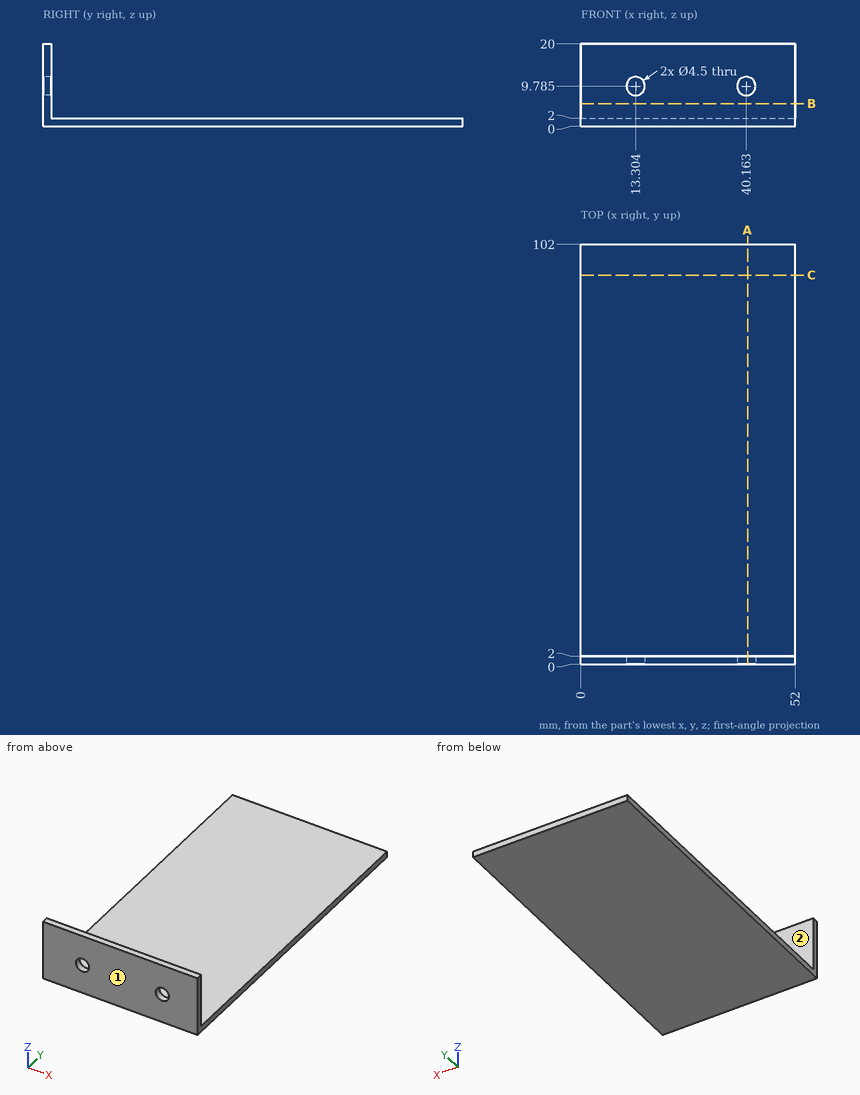
Design review of the part shown in the three views and the two pictorial views. Dimensions are in mm from the part's minimum x, y and z. A direction names the side the tool comes from. Give positions to 0.01 mm unless a question says otherwise; leave off trailing zeros. Loops run counter-clockwise (first coordinate to the right, second up) from the corner with the lowest first, then second, coordinate; pieces in that order, holes last. Notation, with made-up numbers: (8, 6) -> (17, 6) arc R19 ccw to (17, 26) -> close; hole circle Ø4 at (88.25, 33.25). An arc over 180 degrees is marked (long way). One line per item, written item: value.
Q1. We need section A-A on x = 40.5. Give the boundary of the cut face in (y, z), and give its area (3 significant figures).
Numbers:
outline: (0, 0) -> (102, 0) -> (102, 2) -> (2, 2) -> (2, 7.56) -> (0, 7.56) -> close; (0, 12.01) -> (2, 12.01) -> (2, 20) -> (0, 20) -> close
area: 231 mm^2
Q2. For L1, parallel to Z at x = 30, y = 29.5, list the stretches that pass through material, from the lowest coordinate up.
Numbers:
L1: z = 0 to 2
Q3. We need section B-B on z = 5.5. Give the boundary of the cut face in (x, y), and give its area (3 significant figures).
Numbers:
outline: (0, 0) -> (52, 0) -> (52, 2) -> (0, 2) -> close
area: 104 mm^2
Q4. For pin 1 Ø2 at (x, y) = (17, 18.5) entering from +Z; pin 2 Ø4 at (x, z) = (9.5, 18) entering from +Y, all flat-tipped, find the tip position at first contact; note any pin that passes through.
Numbers:
pin 1: stops at z = 2
pin 2: stops at y = 2
Q5. Machinability: for the marked faces 1 and 2, which of the approach directions +Z, -Z, +X, -X, +Y, -Y give a long, thin tool a straight path to every point of the face, cutting with its end or side? Answer none if there is none.
Numbers:
face 1: +Z, -Z, +X, -X, -Y
face 2: +Z, +X, -X, +Y
